```python
from build123d import *

# Parameters (mm, degrees)
BOSS_EXTRUDE1_DEPTH = 2
EXTRUDE_THIN1_DEPTH = 35
EXTRUDE_THIN3_DEPTH = 10
EXTRUDE_THIN4_DEPTH = 33
BOSS_EXTRUDE4_DEPTH = 33
BOSS_EXTRUDE5_DEPTH = 33
SKETCH12_R          = 5
BOSS_EXTRUDE7_DEPTH = 33
SKETCH13_W          = 20
SKETCH13_H          = 20
BOSS_EXTRUDE8_DEPTH = 15
CUT_EXTRUDE1_DEPTH  = 28
CHAMFER2_SIZE       = 5
SKETCH17_R          = 5
BOSS_EXTRUDE9_DEPTH = 33


with BuildPart() as part:
    # Sketch1 → Boss-Extrude1 (new body)
    with BuildSketch(Plane(origin=(0, 0, 0), x_dir=(1, 0, 0), z_dir=(0, 1, 0))):
        with BuildLine():
            Line((-30, 54.486236794), (-30, 55))
            ThreePointArc((-30, 55), (-27.803300859, 60.303300859), (-22.5, 62.5))
            Line((-22.5, 62.5), (22.5, 62.5))
            ThreePointArc((22.5, 62.5), (27.803300859, 60.303300859), (30, 55))
            Line((30, 55), (30, 54.486236794))
            ThreePointArc((30, 54.486236794), (31.846662289, 49.557771239), (36.477272727, 47.056295413))
            ThreePointArc((36.477272727, 47.056295413), (77.388944028, -3.246226107), (30, -47.5))
            Line((30, -47.5), (-30, -47.5))
            ThreePointArc((-30, -47.5), (-77.388944028, -3.246226107), (-36.477272727, 47.056295413))
            ThreePointArc((-36.477272727, 47.056295413), (-31.846662289, 49.557771239), (-30, 54.486236794))
        make_face()
        with BuildLine():
            Line((-30, 32.5), (-10, 32.5))
            Line((-10, 32.5), (-10, -32.5))
            Line((-10, -32.5), (-30, -32.5))
            ThreePointArc((-30, -32.5), (-62.5, 0), (-30, 32.5))
        make_face(mode=Mode.SUBTRACT)
        with BuildLine():
            Line((10, 32.5), (30, 32.5))
            ThreePointArc((30, 32.5), (62.5, 0), (30, -32.5))
            Line((30, -32.5), (10, -32.5))
            Line((10, -32.5), (10, 32.5))
        make_face(mode=Mode.SUBTRACT)
    extrude(amount=BOSS_EXTRUDE1_DEPTH)

    # Sketch2 → Extrude-Thin1 (add)
    with BuildSketch(Plane(origin=(0, 2, 0), x_dir=(1, 0, 0), z_dir=(0, 1, 0))):
        with BuildLine():
            Line((-30, -47.5), (30, -47.5))
            ThreePointArc((30, -47.5), (77.388944028, -3.246226107), (36.477272727, 47.056295413))
            ThreePointArc((36.477272727, 47.056295413), (31.846662289, 49.557771239), (30, 54.486236794))
            Line((30, 54.486236794), (30, 55))
            ThreePointArc((30, 55), (27.803300859, 60.303300859), (22.5, 62.5))
            Line((22.5, 62.5), (-22.5, 62.5))
            ThreePointArc((-22.5, 62.5), (-27.803300859, 60.303300859), (-30, 55))
            Line((-30, 55), (-30, 54.486236794))
            ThreePointArc((-30, 54.486236794), (-31.846662289, 49.557771239), (-36.477272727, 47.056295413))
            ThreePointArc((-36.477272727, 47.056295413), (-77.388944028, -3.246226107), (-30, -47.5))
        make_face()
        with BuildLine():
            Line((-30, -46.5), (30, -46.5))
            ThreePointArc((30, -46.5), (76.391282048, -3.177884504), (36.340909091, 46.065636562))
            ThreePointArc((36.340909091, 46.065636562), (31.092883928, 48.900642499), (29, 54.486236794))
            Line((29, 54.486236794), (29, 55))
            ThreePointArc((29, 55), (27.096194078, 59.596194078), (22.5, 61.5))
            Line((22.5, 61.5), (-22.5, 61.5))
            ThreePointArc((-22.5, 61.5), (-27.096194078, 59.596194078), (-29, 55))
            Line((-29, 55), (-29, 54.486236794))
            ThreePointArc((-29, 54.486236794), (-31.092883928, 48.900642499), (-36.340909091, 46.065636562))
            ThreePointArc((-36.340909091, 46.065636562), (-76.391282048, -3.177884504), (-30, -46.5))
        make_face(mode=Mode.SUBTRACT)
    extrude(amount=EXTRUDE_THIN1_DEPTH)

    # Sketch5 → Extrude-Thin3 (add)
    with BuildSketch(Plane(origin=(0, 2, 0), x_dir=(1, 0, 0), z_dir=(0, 1, 0))):
        with BuildLine():
            Line((30, -34.5), (8, -34.5))
            Line((8, -34.5), (8, 34.5))
            Line((8, 34.5), (30, 34.5))
            ThreePointArc((30, 34.5), (64.5, 0), (30, -34.5))
        make_face()
        with BuildLine():
            Line((30, -32.5), (10, -32.5))
            Line((10, -32.5), (10, 32.5))
            Line((10, 32.5), (30, 32.5))
            ThreePointArc((30, 32.5), (62.5, 0), (30, -32.5))
        make_face(mode=Mode.SUBTRACT)
    extrude_thin3 = extrude(amount=EXTRUDE_THIN3_DEPTH)

    # Mirror1: Extrude-Thin3 across plane
    add(extrude_thin3.mirror(Plane(origin=(0, 0, 0), x_dir=(0, 0, 1), z_dir=(1, 0, 0))))

    # Sketch6 → Extrude-Thin4 (add)
    with BuildSketch(Plane(origin=(0, 2, 0), x_dir=(1, 0, 0), z_dir=(0, 1, 0))):
        with BuildLine():
            Line((-30, -46.5), (30, -46.5))
            ThreePointArc((30, -46.5), (76.391282048, -3.177884504), (36.340909091, 46.065636562))
            ThreePointArc((36.340909091, 46.065636562), (31.092883928, 48.900642499), (29, 54.486236794))
            Line((29, 54.486236794), (29, 55))
            ThreePointArc((29, 55), (27.096194078, 59.596194078), (22.5, 61.5))
            Line((22.5, 61.5), (-22.5, 61.5))
            ThreePointArc((-22.5, 61.5), (-27.096194078, 59.596194078), (-29, 55))
            Line((-29, 55), (-29, 54.486236794))
            ThreePointArc((-29, 54.486236794), (-31.092883928, 48.900642499), (-36.340909091, 46.065636562))
            ThreePointArc((-36.340909091, 46.065636562), (-76.391282048, -3.177884504), (-30, -46.5))
        make_face()
        with BuildLine():
            Line((-30, -45), (30, -45))
            ThreePointArc((30, -45), (74.894789079, -3.075372101), (36.136363636, 44.579648286))
            ThreePointArc((36.136363636, 44.579648286), (29.962216386, 47.914949388), (27.5, 54.486236794))
            Line((27.5, 54.486236794), (27.5, 55))
            ThreePointArc((27.5, 55), (26.035533906, 58.535533906), (22.5, 60))
            Line((22.5, 60), (-22.5, 60))
            ThreePointArc((-22.5, 60), (-26.035533906, 58.535533906), (-27.5, 55))
            Line((-27.5, 55), (-27.5, 54.486236794))
            ThreePointArc((-27.5, 54.486236794), (-29.962216386, 47.914949388), (-36.136363636, 44.579648286))
            ThreePointArc((-36.136363636, 44.579648286), (-74.894789079, -3.075372101), (-30, -45))
        make_face(mode=Mode.SUBTRACT)
    extrude(amount=EXTRUDE_THIN4_DEPTH)

    # Sketch8 → Boss-Extrude4 (add)
    with BuildSketch(Plane(origin=(0, 2, 0), x_dir=(1, 0, 0), z_dir=(0, 1, 0))):
        with BuildLine():
            ThreePointArc((-74.464958868, 6.918629407), (-68.060713157, 0), (-74.464958868, -6.918629407))
            ThreePointArc((-74.464958868, -6.918629407), (-75, 0), (-74.464958868, 6.918629407))
        make_face()
    boss_extrude4 = extrude(amount=BOSS_EXTRUDE4_DEPTH)

    # Mirror2: Boss-Extrude4 across plane
    add(boss_extrude4.mirror(Plane(origin=(0, 0, 0), x_dir=(0, 0, 1), z_dir=(1, 0, 0))))

    # Sketch9 → Boss-Extrude5 (add)
    with BuildSketch(Plane(origin=(0, 2, 0), x_dir=(1, 0, 0), z_dir=(0, 1, 0))):
        with BuildLine():
            Line((8, -45), (-8, -45))
            ThreePointArc((-8, -45), (0, -37), (8, -45))
        make_face()
    extrude(amount=BOSS_EXTRUDE5_DEPTH)

    # Sketch12 → Boss-Extrude7 (add)
    with BuildSketch(Plane(origin=(0, 2, 0), x_dir=(1, 0, 0), z_dir=(0, 1, 0))):
        with Locations((-22.5, 55)):
            Circle(SKETCH12_R)
        with Locations((22.5, 55)):
            Circle(SKETCH12_R)
    extrude(amount=BOSS_EXTRUDE7_DEPTH)

    # Sketch13 → Boss-Extrude8 (add)
    with BuildSketch(Plane(origin=(0, 2, 0), x_dir=(1, 0, 0), z_dir=(0, 1, 0))):
        with Locations((0, 50)):
            Rectangle(SKETCH13_W, SKETCH13_H)
    extrude(amount=BOSS_EXTRUDE8_DEPTH)

    # Sketch14 → Cut-Extrude1 (cut)
    with BuildSketch(Plane.XY.offset(-40)):
        Polygon((5.773502692, 9.5), (2.886751346, 14.5), (-2.886751346, 14.5), (-5.773502692, 9.5), (-2.886751346, 4.5), (2.886751346, 4.5), align=None)
    extrude(amount=-CUT_EXTRUDE1_DEPTH, mode=Mode.SUBTRACT)

    # Chamfer2
    chamfer2_edges = [part.edges().sort_by_distance(p)[0] for p in [
        (10, 17, -50),
        (-10, 17, -50),
    ]]
    chamfer(chamfer2_edges, length=CHAMFER2_SIZE)

    # Sketch17 → Boss-Extrude9 (add)
    with BuildSketch(Plane(origin=(0, 2, 0), x_dir=(1, 0, 0), z_dir=(0, 1, 0))):
        Circle(SKETCH17_R)
    extrude(amount=BOSS_EXTRUDE9_DEPTH)


solid = part.part
```
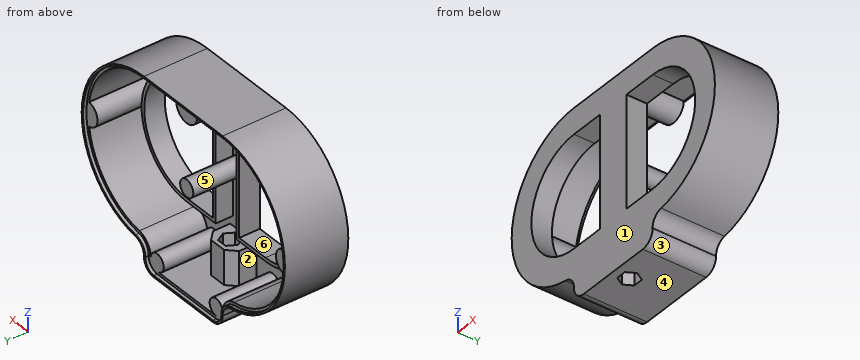
Part model, mm, in its own coordinate system. Face numbers are marked on the shaded views. A direction names the side the tool comes from. Round coordinates to 2 decimals unless told otherwise and drop trailing zeros. Loops run counter-clockwise (first coordinate to the right, second up) from the corner with the lowest first, then second, coordinate; pieces in that order, holes last. Notation, with made-up numbers: (-1, 60.5) -> (20, 60.5) arc R20 cw to (20, 86.5) -> close; hole circle Ø8 at (40.25, -15). An arc over 180 degrees is marked (long way). Use one line per item in the form item = value. Start each with the question number.
Item 1: Tool access for the marked faces 4, 5 and 6: list every direction of +Z, -Z, +X, -X, +Y, -Y with a clear straight run to the whole face (end or side of a thin tool).
Item 2: Band-saw the part on A-A (z = 0). Give the number of separate pieces and of enclosed holes in the cut face, plus the area to 3 significant figures.
Item 3: Drill centre lines: line 1 along X through (y, z) = (23.5, 1.5); line 2 along X through (y, z) = (32.5, -2.5); line 3 along Z through (x, y) = (32, 6). Where is each one in solid material? Low to high.
Item 4: Drop flat-ended pins along their axis: pin 1 Ø2 at (x, z) = (-57, 30.5) entering from -Y; pin 2 Ø1.5 at (y, z) = (33, 31) entering from -X; pin 3 Ø3 at (y, z) = (4.5, -10.5) entering from -X; pin 4 Ø6 at (y, z) = (33, -6.5) entering from -X. Give the stop position or say it passes through.
Item 5: Band-saw the part on D-D (z = 40.5). List the corners of the cut face in (x, y), plus the area to 3 significant figures.
Item 6: Band-saw the part on C-C (x = -43.5). List the corners of the cut face in (y, z).
Item 7: Two-plate mould, pull along X, no slides. Class the marked faces 1, 2 and 3: released by +X, released by -X, zero draft, split by the parting line, or undercut.
Item 8: Band-saw the part on B-B (y = 31). List the corners of the cut face in (x, z), plus the area to 3 significant figures.
Data:
q1.face_4 = -Z, +X, -X, +Y, -Y
q1.face_5 = +Y
q1.face_6 = +Y, -Y
q2.separate_pieces = 3
q2.enclosed_holes = 0
q2.area = 1,140 mm^2
q3.line_1 = -77.48 to -68.22, -4.77 to 4.77, 68.22 to 77.48
q3.line_2 = -77.43 to -68.53, -4.33 to 4.33, 68.53 to 77.43
q3.line_3 = -49.39 to -46.13, -34.44 to -32.44, 32.44 to 34.44, 44.96 to 47.46
q4.pin_1 = 0
q4.pin_2 = -66.62
q4.pin_3 = -76.64
q4.pin_4 = -77.37
q5.outline = (-54.82, 0) -> (54.82, 0) -> (54.82, 37) -> (52.85, 37) -> (52.85, 35) -> (49.62, 35) -> (49.62, 2) -> (6.61, 2) -> (6.61, 35) -> (-6.61, 35) -> (-6.61, 2) -> (-49.62, 2) -> (-49.62, 35) -> (-52.85, 35) -> (-52.85, 37) -> (-54.82, 37) -> close
q5.area = 1,010 mm^2
q6.outline = (0, -45.54) -> (37, -45.54) -> (37, -44.5) -> (35, -44.5) -> (35, -42.93) -> (2, -42.93) -> (2, -31.75) -> (12, -31.75) -> (12, -29.56) -> (0, -29.56) -> close; (0, 29.56) -> (12, 29.56) -> (12, 31.75) -> (2, 31.75) -> (2, 42.93) -> (35, 42.93) -> (35, 44.5) -> (37, 44.5) -> (37, 45.54) -> (0, 45.54) -> close
q7.face_1 = zero draft
q7.face_2 = undercut
q7.face_3 = released by +X
q8.outline = (-36.48, -47.06) arc R7.5 cw to (-30, -54.49) -> (-30, -55) arc R7.5 ccw to (-22.5, -62.5) -> (22.5, -62.5) arc R7.5 ccw to (30, -55) -> (30, -54.49) arc R7.5 cw to (36.48, -47.06) arc R47.5 ccw to (30, 47.5) -> (-30, 47.5) arc R47.5 ccw to start; circle Ø10 at (0, 0); hole (-74.46, -6.92) arc R45 ccw to (-36.14, -44.58) arc R10 cw to (-27.5, -54.49) -> (-27.5, -55) arc R5 cw (long way) to (-22.5, -60) -> (22.5, -60) arc R5 cw (long way) to (27.5, -55) -> (27.5, -54.49) arc R10 cw to (36.14, -44.58) arc R45 ccw to (74.46, -6.92) arc R6.94 cw to (74.46, 6.92) arc R45 ccw to (30, 45) -> (8, 45) arc R8 cw to (-8, 45) -> (-30, 45) arc R45 ccw to (-74.46, 6.92) arc R6.94 cw to start
q8.area = 1,550 mm^2
